Autodesk Inventor part; units mm, degrees
ref_plane "YZ Plane" through (0, 0, 0) normal (1, 0, 0) x (0, 1, 0)
ref_plane "XZ Plane" through (0, 0, 0) normal (0, 1, 0) x (-1, 0, 0)
ref_plane "XY Plane" through (0, 0, 0) normal (0, 0, 1) x (1, 0, 0)
sketch "스케치1" plane through (0, 0, 0) normal (0, 0, 1) x (1, 0, 0)
  line L0 (0, 0) -> (47.183, 0)
  line L1 (47.183, 0) -> (47.183, -4)
  line L2 (47.183, -4) -> (0, -4)
  line L3 (0, -4) -> (0, 0)
  line L4 (47.183, -4) -> (51.183, -4)
  line L5 (51.183, -4) -> (51.183, 31.431)
  line L6 (51.183, 31.431) -> (47.183, 31.431)
  line L7 (47.183, 31.431) -> (47.183, -4)
  point P0 (47.183, 0)
  dimension "d0" = 47.183
  dimension "d1" = 31.431
  dimension "d2" = 4
  dimension "d3" = 4
extrude "돌출1" add sketch "스케치1" along normal blind 10
sketch "스케치2" plane through (0, 0, 0) normal (0, 1, 0) x (1, 0, 0)
  line L0 (0, 0) -> (0, -10)
  line L1 (0, -5) -> (47.183, -5) construction
  line L2 (47.183, 0) -> (47.183, -10)
  circle A0 centre (23.5915, -5) radius 2.5
  dimension "d6" = 5
extrude "돌출2" cut sketch "스케치2" against normal blind 9.25
sketch "스케치3" plane through (47.183, 0, 0) normal (-1, 0, 0) x (0, 0, 1)
  line L0 (0, 31.431) -> (10, 31.431)
  line L1 (5, 31.431) -> (5, 4.931)
  circle A0 centre (5, 18.181) radius 2.5
  point P0 (0, 0)
  dimension "d9" = 5
extrude "돌출3" cut sketch "스케치3" against normal blind 8.75
properties part number "베벨기어 003"
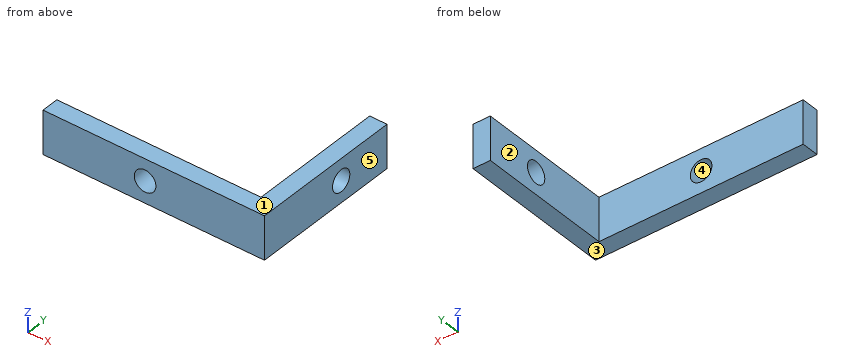
Source: CAD feature listing. Evaluate the final solid. Frame: model axes, mm. Face numbers are marked on the shaded views. A direction names the side the tool comes from. Coordinates: 2 decimals unless noted, no trailing zeros. Write each loop counter-clockwise with the first axis right and the second up, starting at its lowest first coordinate (ties: lowest second). Pieces come first, ordered by that corner, then holes. Notation, with made-up numbers: (-16, 2) - (41, 2) arc R21 ccw to (41, 32) - close; hole circle Ø11 at (73.5, 61.25). An arc over 180 degrees is marked (long way). Answer as a JSON object with one key per item and string values.
Q1. Draft query along Z for the marked faces 3, 4 and 5. Return one class per face: released by +Z, released by -Z, zero draft, split by the parting line, or undercut.
Ans:
{"face 3": "released by -Z", "face 4": "undercut", "face 5": "zero draft"}
Q2. Material intervals for line 1 (X direction, y = -3, z = 5); line 2 (Y direction, x = 49, z = 5); line 3 (X direction, y = 3.5, z = 1.25), sorted ascending. Write a range as [from, to].
Ans:
{"line 1": "x = [0, 21.09], [26.09, 51.18]", "line 2": "y = [-4, 15.68], [20.68, 31.43]", "line 3": "x = [47.18, 51.18]"}
Q3. Section query A-A, the plane z = 5. Output: boundary loops of the cut face in (x, y), plus the area to 3 significant figures.
Ans:
{"outline": "(0, -4) - (21.09, -4) - (21.09, 0) - (0, 0) - close; (26.09, -4) - (51.18, -4) - (51.18, 15.68) - (47.18, 15.68) - (47.18, 0) - (26.09, 0) - close; (47.18, 20.68) - (51.18, 20.68) - (51.18, 31.43) - (47.18, 31.43) - close", "area": "290 mm2"}
Q4. Section query B-B, the plane x = 22. Output: boundary loops of the cut face in (y, z), plus the area to 3 significant figures.
Ans:
{"outline": "(-4, 0) - (0, 0) - (0, 3.07) - (-4, 3.07) - close; (-4, 6.93) - (0, 6.93) - (0, 10) - (-4, 10) - close", "area": "24.6 mm2"}
Q5. Section query D-D, the plane y = 27. Output: boundary loops of the cut face in (x, z).
Ans:
{"outline": "(47.18, 0) - (51.18, 0) - (51.18, 10) - (47.18, 10) - close"}
Q6. Section query C-C, the plane y = -1. Output: boundary loops of the cut face in (x, z), plus the area to 3 significant figures.
Ans:
{"outline": "(0, 0) - (51.18, 0) - (51.18, 10) - (0, 10) - close; hole circle Ø5 at (23.59, 5)", "area": "492 mm2"}
Q7. First-contact query: pin 1 Ø3 at (x, z) = (27.5, 5) entering from +Y; pin 2 Ø1 at (x, y) = (45.5, 9.5) entering from -Z; pin 3 Ø1 at (y, z) = (18, 1.5) entering from -X. Flat tips, straight axial feed; report the tip coordinate or a pass-through.
Ans:
{"pin 1": "stops at y = 0", "pin 2": "passes through", "pin 3": "stops at x = 47.18"}
Q8. Set-up query: the marked faces 1 and 2. Return all of +Z, -Z, +X, -X, +Y, -Y with unobstructed straight access to the full face (end or side cutting, diameter ignored); none if empty.
Ans:
{"face 1": "+Z, +X, -X, +Y, -Y", "face 2": "+Z, -Z, -X, +Y"}
